The figure shows three views and two pictorial views of one solid part (mm, origin at its lowest corner). Answer the questions. Give positions to 0.01 mm unless a question says otherwise; leave off trailing zeros. Loops run counter-clockwise (first coordinate to the right, second up) from the corner with the lowest first, then second, coordinate; pieces in that order, holes last. Notation, with made-up numbers: (59, 60.5) -> (74, 60.5) arc R26 ccw to (74, 80.5) -> close; hole circle Ø8 at (23.25, 52.5). An arc over 180 degrees is marked (long way). Answer as CSV lines item,"result". Start each with the question number.
1. A flat-ended cylindrical pin translates along its axis: pin 1 Ø3 at (x, y) = (131.5, 201) entering from +Z. Find the tip coordinate at first contact, or state that the pin passes through.
2. Find section B-B, the plane y = 240. Give the vertices of the cut face in (x, z), and give its area (3 significant figures).
3. Find the intervals of material crossed by line 1 along Y through (x, z) = (235, 3); line 2 along X through (y, z) = (267, 17.5); line 3 along Y through (x, z) = (221, 11.5), in increasing order.
4. Find section A-A, the plane z = 6.5. Give the vertices of the cut face in (x, y), and give its area (3 significant figures).
5. Find section D-D, the plane x = 150. Give the vertices of the cut face in (y, z).
6. Find section C-C, the plane x = 235. Give the vertices of the cut face in (y, z).
7. Determine the mould class of the marked faces 1 and 2 for opening direction Y: +Y half, -Y half, draft (parallel to the pull), parting line (faces both ways), or undercut.
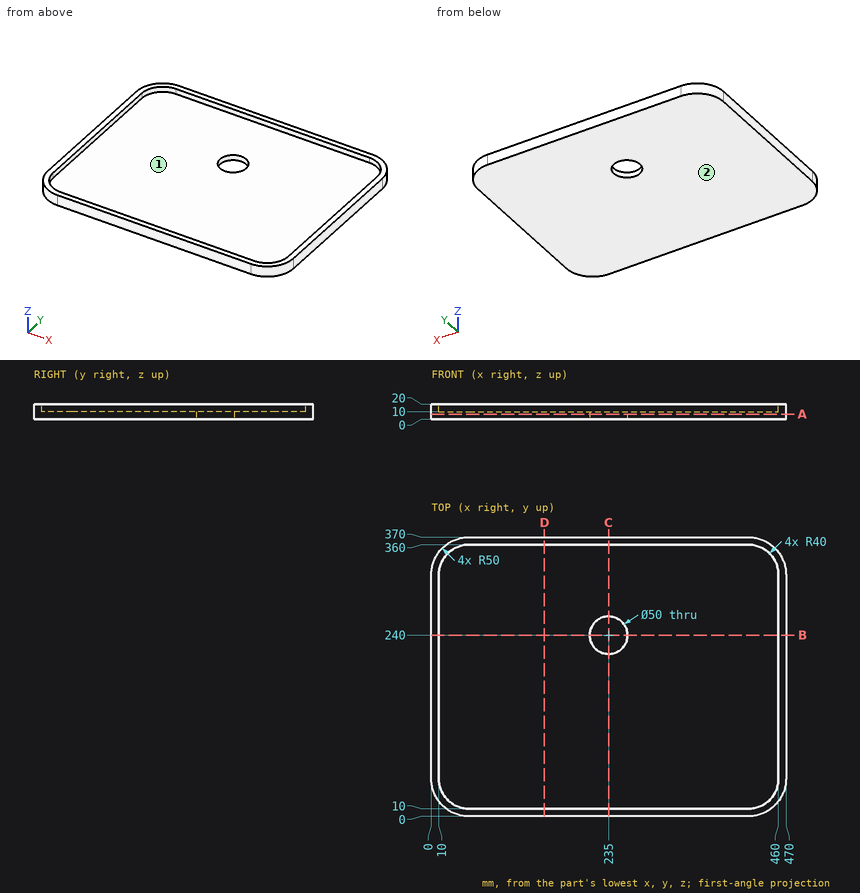
Resolved:
1,pin 1,"stops at z = 10"
2,outline,"(0, 0) -> (210, 0) -> (210, 10) -> (10, 10) -> (10, 20) -> (0, 20) -> close; (260, 0) -> (470, 0) -> (470, 20) -> (460, 20) -> (460, 10) -> (260, 10) -> close"
2,area,"4,400 mm^2"
3,line 1,"y = 0 to 215, 265 to 370"
3,line 2,"x = 0 to 10, 460 to 470"
3,line 3,"y = 0 to 10, 360 to 370"
4,outline,"(0, 50) arc R50 ccw to (50, 0) -> (420, 0) arc R50 ccw to (470, 50) -> (470, 320) arc R50 ccw to (420, 370) -> (50, 370) arc R50 ccw to (0, 320) -> close; hole circle Ø50 at (235, 240)"
4,area,"170,000 mm^2"
5,outline,"(0, 0) -> (370, 0) -> (370, 20) -> (360, 20) -> (360, 10) -> (10, 10) -> (10, 20) -> (0, 20) -> close"
6,outline,"(0, 0) -> (215, 0) -> (215, 10) -> (10, 10) -> (10, 20) -> (0, 20) -> close; (265, 0) -> (370, 0) -> (370, 20) -> (360, 20) -> (360, 10) -> (265, 10) -> close"
7,face 1,"undercut"
7,face 2,"draft"
